from build123d import *

# Parameters (mm, degrees)
SKETCH018_W             = 125
SKETCH018_H             = 55.88
SKETCH018_R             = 1.5875
PAD007_DEPTH            = 1.5
SKETCH017_W             = 26
SKETCH017_H             = 5
PAD008_DEPTH            = 8.85
SKETCH019_W             = 16.4
SKETCH019_H             = 16
PAD009_DEPTH            = 12
BODY004_PLACEMENT_ANGLE = 90


with BuildPart() as part:
    # Sketch018 → Pad007 (new body)
    with BuildSketch(Plane.XY):
        with Locations((62.5, 27.94)):
            Rectangle(SKETCH018_W, SKETCH018_H)
        with Locations((21.59, 16.51)):
            Circle(SKETCH018_R, mode=Mode.SUBTRACT)
        with Locations((83.55, 52.07)):
            Circle(SKETCH018_R, mode=Mode.SUBTRACT)
        with Locations((96, 21.57)):
            Circle(SKETCH018_R, mode=Mode.SUBTRACT)
    extrude(amount=PAD007_DEPTH)

    # Sketch017 (on Face8 of Pad007) → Pad008 (join, symmetric)
    with BuildSketch(Plane(origin=(0, 0, 0), x_dir=(1, 0, 0), z_dir=(0, 0, -1))):
        with Locations((49, -10.38)):
            Rectangle(SKETCH017_W, SKETCH017_H)
        with Locations((112, -10.38)):
            Rectangle(SKETCH017_W, SKETCH017_H)
        with Locations((112, -53.38)):
            Rectangle(SKETCH017_W, SKETCH017_H)
        with Locations((49, -53.38)):
            Rectangle(SKETCH017_W, SKETCH017_H)
    extrude(amount=PAD008_DEPTH, both=True)

    # Sketch019 (on Face4 of Pad008) → Pad009 (join)
    with BuildSketch(Plane.XY.offset(1.5)):
        with Locations((7.2, 46.68)):
            Rectangle(SKETCH019_W, SKETCH019_H)
    extrude(amount=PAD009_DEPTH)


with BuildPart() as part_1:
    # Body004 placement: moved
    add(part.part.moved(Location((28, 0, 39))).rotate(Axis((28, 0, 39), (0, 0, 1)), BODY004_PLACEMENT_ANGLE))


solid = part_1.part
The model under review builds one solid part; all positions refer to its coordinate system, in mm. A direction names the side the tool comes from. Coordinates: 2 decimals unless noted, no trailing zeros. Loops run counter-clockwise (first coordinate to the right, second up) from the corner with the lowest first, then second, coordinate; pieces in that order, holes last.
(1) Consider section C-C, the plane y = 83.55. Give the boundary of the cut face in (x, z).
Determined:
outline: (-27.88, 39) - (-25.66, 39) - (-25.66, 40.5) - (-27.88, 40.5) - close; (-22.48, 39) - (28, 39) - (28, 40.5) - (-22.48, 40.5) - close
(2) Consider section D-D, the plane y = 102. Give the boundary of the cut face in (x, z).
Determined:
outline: (-27.88, 30.15) - (-22.88, 30.15) - (-22.88, 39) - (15.12, 39) - (15.12, 30.15) - (20.12, 30.15) - (20.12, 39) - (28, 39) - (28, 40.5) - (20.12, 40.5) - (20.12, 47.85) - (15.12, 47.85) - (15.12, 40.5) - (-22.88, 40.5) - (-22.88, 47.85) - (-27.88, 47.85) - close
(3) Consider section B-B, the plane x = 6.43. Give the boundary of the cut face in (y, z).
Determined:
outline: (0, 39) - (94.41, 39) - (94.41, 40.5) - (0, 40.5) - close; (97.59, 39) - (125, 39) - (125, 40.5) - (97.59, 40.5) - close
(4) Draft analysis for pull direction Y (two halves, no side actions). For faces 1 (the cylindrical face through (6.36, 94.414, 39.74)), 2 (the flat face through (-25, 49, 47.85)), state which applies: +Y half, -Y half, draft (parallel to the pull), parting line (faces both ways), or undercut.
Determined:
face 1: undercut
face 2: draft
(5) Consider section A-A, the plane z = 45. Give the boundary of the cut face in (x, y), plus the area to 3 significant figures.
Determined:
outline: (-27.88, 36) - (-22.88, 36) - (-22.88, 62) - (-27.88, 62) - close; (-27.88, 99) - (-22.88, 99) - (-22.88, 125) - (-27.88, 125) - close; (-26.68, -1) - (-10.68, -1) - (-10.68, 15.4) - (-26.68, 15.4) - close; (15.12, 36) - (20.12, 36) - (20.12, 62) - (15.12, 62) - close; (15.12, 99) - (20.12, 99) - (20.12, 125) - (15.12, 125) - close
area: 782 mm2
(6) Wall thickness on L1, parallel to X at y = 108, z = 40.75; L2, parallel to X at y = 21.59, z = 40.05; L3, parallel to Y at x = -24.07, z = 39.85: over which ranges is each line inside the solid? List them lowest first.
Determined:
L1: x = -27.88 to -22.88, 15.12 to 20.12
L2: x = -27.88 to 9.9, 13.08 to 28
L3: y = 0 to 81.96, 85.14 to 125
(7) Insertion check: P1, Ø1.6, axis at x = 4, z = 40, coming from the -Y side; P2, Ø2.5, axis at y = 105.5, z = 35, coming from the +X side; P3, Ø4, axis at x = -17, y = 47.5, coming from the +Z side. Each pin has a flat end and moves straight along its axis. Give the tip position at first contact, or say it passes through.
Determined:
P1: stops at y = 0
P2: stops at x = 20.12
P3: stops at z = 40.5
(8) Tool access review of faces 3 (the flat face through (18, 62, 35)), 4 (the flat face through (15.12, 49, 44)), 5 (the flat face through (15.12, 49, 35)), 6 (the flat face through (20.12, 112, 35)): name each direction out of +Z, -Z, +X, -X, +Y, -Y from which nothing blocks a thin tool from reaching the whole face with its end or side.
Determined:
face 3: -Z, +X, -X
face 4: +Z, +Y, -Y
face 5: -Z, +Y, -Y
face 6: -Z, +X, +Y, -Y
